from build123d import *

# Parameters (mm, degrees)
ESQUISSE1_W       = 10
ESQUISSE1_H       = 0.8
R_VOLUTION1_ANGLE = 355
CHANFREIN1_SIZE   = 0.5


with BuildPart() as part:
    # Esquisse1 → Révolution1 (revolve)
    with BuildSketch(Plane.XY):
        with Locations((0, 3.6)):
            Rectangle(ESQUISSE1_W, ESQUISSE1_H)
    revolve(axis=Axis((-7.531341075, 0, 0), (1, 0, 0)), revolution_arc=R_VOLUTION1_ANGLE)

    # Chanfrein1
    chanfrein1_edges = [part.edges().sort_by_distance(p)[0] for p in [
        (5, -3.996192886, 0.174477549),
        (-5, -3.996192886, 0.174477549),
    ]]
    chamfer(chanfrein1_edges, length=CHANFREIN1_SIZE)


solid = part.part
Check sheet for the modelled part. Datum: model origin and axes. Units: mm. Give positions to 0.01 mm unless a question says otherwise; leave off trailing zeros. Write each loop counter-clockwise with the first axis right and the second up, starting at its lowest first coordinate (ties: lowest second). Pieces come first, ordered by that corner, then holes. Notation, with made-up numbers: (74, 37) -> (101, 37) arc R29 ccw to (101, 67) -> close; hole circle Ø2 at (-26.75, 27.25). An arc over 180 degrees is marked (long way). Use one line per item in the form item = value. Start each with the question number.
1. Thickness scan on line 1 along Z through (x, y) = (-1.5, 0); line 2 along Z through (x, y) = (0.25, -1); line 3 along Y through (x, z) = (3.5, 2.5). Record the ranges inside material, lowest first. Write a range as from..to.
2. Mould release check, pull along Z, two halves, no side actions. Record for faces 1 (the flat face through (-0.1, 3.6, 0)), 2 (the cylindrical face through (0, -4, 0)): pulls with the +Z half, pulls with the -Z half, needs draft (parallel to the pull), parting line crosses it, or undercut.
3. Section check A-A (y = 0). Record the cut outline in (x, z).
4. Section check B-B (x = -2.75). Record the cut outline in (y, z), and give its area (3 significant figures).
5. Go/stop test with flat-tipped pins: P1, Ø3, axis at x = 3, y = 3, coming from the +Z side; P2, Ø4, axis at y = 0, z = 0, coming from the +X side; P3, Ø1, axis at x = -1.5, z = -2, coming from the +Y side; P4, Ø2, axis at x = 0, y = 3, coming from the -Z side. Record where each tip stops, or that it passes through.
Conclusion:
q1.line_1 = -4..-3.2, 3.2..4
q1.line_2 = -3.87..-3.04, 3.04..3.87
q1.line_3 = -3.12..-2, 2..3.12
q2.face_1 = undercut
q2.face_2 = parting line crosses it
q3.outline = (-5, -3.5) -> (-4.5, -4) -> (4.5, -4) -> (5, -3.5) -> (5, -3.2) -> (-5, -3.2) -> close; (-5, 3.2) -> (5, 3.2) -> (5, 3.5) -> (4.5, 4) -> (-4.5, 4) -> (-5, 3.5) -> close
q4.outline = (3.19, -0.28) arc R3.2 cw (long way) to (3.2, 0) -> (4, 0) arc R4 ccw (long way) to (3.98, -0.35) -> close
q4.area = 17.8 mm²
q5.P1 = 3.71
q5.P2 = through
q5.P3 = 3.71
q5.P4 = -3.46
